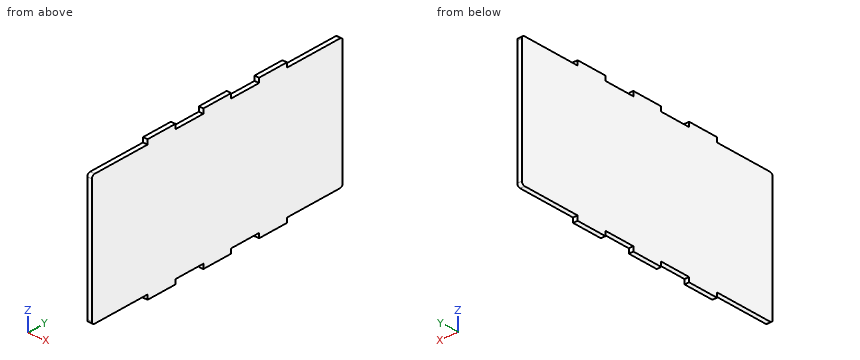
from build123d import *

# Parameters (mm, degrees)
SKETCH1_W           = 3
SKETCH1_H           = 180
EXTRUDE_THIN1_DEPTH = 90
CAVITY1_START       = -65.602294015
CAVITY1_OUTLINE_W   = 3
CAVITY1_OUTLINE_H   = 3
CAVITY1_DEPTH       = 40
CAVITY1_START_2     = 74.397705985
CAVITY1_2_OUTLINE_W = 3
CAVITY1_2_OUTLINE_H = 3
CAVITY1_2_DEPTH     = 40
CAVITY1_START_3     = -5.602294015
CAVITY1_3_OUTLINE_W = 3
CAVITY1_3_OUTLINE_H = 3
CAVITY1_3_DEPTH     = 20
CAVITY1_START_4     = 34.397705985
CAVITY1_4_OUTLINE_W = 3
CAVITY1_4_OUTLINE_H = 3
CAVITY1_4_DEPTH     = 20
FILLET1_R           = 2


# Read off the part's stored shape, not the designer's step: Cavity1
with BuildPart() as part:
    # Sketch1 → Extrude-Thin1 (new body)
    with BuildSketch(Plane.XY.offset(1.5)):
        with Locations((-92.414893617, 24.397705985)):
            Rectangle(SKETCH1_W, SKETCH1_H)
    extrude(amount=-EXTRUDE_THIN1_DEPTH)

    # Cavity1 outline → Cavity1 (cut)
    with BuildSketch(Plane(origin=(0, 0, 0), x_dir=(1, 0, 0), z_dir=(0, 1, 0)).offset(CAVITY1_START)):
        with Locations((-92.414893617, 87)):
            Rectangle(CAVITY1_OUTLINE_W, CAVITY1_OUTLINE_H)
        with Locations((-92.414893617, 0)):
            Rectangle(CAVITY1_OUTLINE_W, CAVITY1_OUTLINE_H)
    extrude(amount=CAVITY1_DEPTH, mode=Mode.SUBTRACT)

    # Cavity1 2 outline → Cavity1 2 (cut)
    with BuildSketch(Plane(origin=(0, 0, 0), x_dir=(1, 0, 0), z_dir=(0, 1, 0)).offset(CAVITY1_START_2)):
        with Locations((-92.414893617, 87)):
            Rectangle(CAVITY1_2_OUTLINE_W, CAVITY1_2_OUTLINE_H)
        with Locations((-92.414893617, 0)):
            Rectangle(CAVITY1_2_OUTLINE_W, CAVITY1_2_OUTLINE_H)
    extrude(amount=CAVITY1_2_DEPTH, mode=Mode.SUBTRACT)

    # Cavity1 3 outline → Cavity1 3 (cut)
    with BuildSketch(Plane(origin=(0, 0, 0), x_dir=(1, 0, 0), z_dir=(0, 1, 0)).offset(CAVITY1_START_3)):
        with Locations((-92.414893617, 87)):
            Rectangle(CAVITY1_3_OUTLINE_W, CAVITY1_3_OUTLINE_H)
        with Locations((-92.414893617, 0)):
            Rectangle(CAVITY1_3_OUTLINE_W, CAVITY1_3_OUTLINE_H)
    extrude(amount=CAVITY1_3_DEPTH, mode=Mode.SUBTRACT)

    # Cavity1 4 outline → Cavity1 4 (cut)
    with BuildSketch(Plane(origin=(0, 0, 0), x_dir=(1, 0, 0), z_dir=(0, 1, 0)).offset(CAVITY1_START_4)):
        with Locations((-92.414893617, 87)):
            Rectangle(CAVITY1_4_OUTLINE_W, CAVITY1_4_OUTLINE_H)
        with Locations((-92.414893617, 0)):
            Rectangle(CAVITY1_4_OUTLINE_W, CAVITY1_4_OUTLINE_H)
    extrude(amount=CAVITY1_4_DEPTH, mode=Mode.SUBTRACT)

    # Fillet1
    fillet1_edges = [part.edges().sort_by_distance(p)[0] for p in [
        (-92.414893617, -65.602294015, -85.5),
        (-92.414893617, 114.397705985, -85.5),
        (-92.414893617, 114.397705985, -1.5),
        (-92.414893617, -65.602294015, -1.5),
    ]]
    fillet(fillet1_edges, radius=FILLET1_R)


solid = part.part
Here's how the part is built. I have some questions about the finished solid (model axes, mm). Coordinates: 2 decimals unless noted, no trailing zeros. Loops run counter-clockwise (first coordinate to the right, second up) from the corner with the lowest first, then second, coordinate; pieces in that order, holes last.
1. I need wall thicknesses on L1, parallel to Z at x = -92.2, y = -36; L2, parallel to Y at x = -92.3, z = -2; L3, parallel to Y at x = -93, z = -84. Which ranges of each line are inside material? Lowest first, please.
2. Imagine slicing it at B-B, the plane y = -40. Please give me the cut outline in (x, z), and give its area (3 significant figures).
3. For P1, Ø0.9, axis at x = -92, y = 95, coming from the +Z side; P2, Ø1.5, axis at x = -92, z = 0, coming from the -Y side; P3, Ø0.9, axis at x = -93, z = 0.5, coming from the +Y side, each with a flat end and sliding along its axis, tell me the tip position at first contact or that it passes through.
Taken from the geometry:
1. L1: z = -85.5 to -1.5
1. L2: y = -64.93 to 113.72
1. L3: y = -65.54 to 114.33
2. outline: (-93.91, -85.5) - (-90.91, -85.5) - (-90.91, -1.5) - (-93.91, -1.5) - close
2. area: 252 mm2
3. P1: stops at z = -1.5
3. P2: stops at y = -25.6
3. P3: stops at y = 74.4
